Can you work these out from the model? Positions are in its coordinate system, mm. Coordinates: 2 decimals unless noted, no trailing zeros. Order: outer loops, then holes, each group sorted by start corner. A loop starts at its lowest first (then second) coordinate and runs counter-clockwise, first axis right, second up. Notation, with made-up numbers: (85.5, -3.75) -> (122.5, -3.75) arc R20 cw to (122.5, 31.25) -> close; hole circle Ø3 at (52.25, 17.25). An arc over 180 degrees is marked (long way). Return JSON: item names as keys, results as strings. Group by question number.
1) If I drill on probe 1 along Z at (x, y) = (0.55, 0); probe 2 along Z at (x, y) = (0.9, -0.75); probe 3 along Z at (x, y) = (0.4, -9.25), over which ranges is the centre line in solid material (lowest first)? Write a range as from..to.
2) If we section it at C-C, the plane y = 9: Please give me the cut outline in (x, z).
3) For pin 1 (1.8 mm diameter, centred on y = -9, z = 0, fed in from +X), with a flat end and sliding along its axis, tell me the tip position at first contact or that it passes through.
4) If we section it at A-A, the plane z = 0: Please give me the cut outline in (x, y).
from build123d import *

# Parameters (mm, degrees)
F0_R     = 11.5
F1_DEPTH = 1
F2_R     = 1
F3_DEPTH = 1.001


with BuildPart() as f1:
    # F0 (on Right) → F1 (new body)
    with BuildSketch(Plane.YZ):
        Circle(F0_R)
    extrude(amount=F1_DEPTH)

    # F2 (on face) → F3 (cut, through all)
    with BuildSketch(Plane.YZ.offset(1)):
        with Locations((0, 9)):
            Circle(F2_R)
        with Locations((9, 0)):
            Circle(F2_R)
        with Locations((0, -9)):
            Circle(F2_R)
        with Locations((-9, 0)):
            Circle(F2_R)
    extrude(amount=-F3_DEPTH, mode=Mode.SUBTRACT)


solid = f1.part
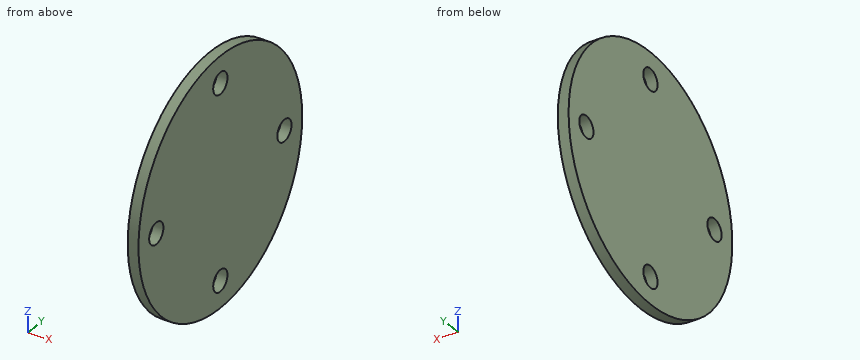
Result sheet:
{
 "1": {"probe 1": "z = -11.5..-10, -8..8, 10..11.5", "probe 2": "z = -11.48..-9.66, -8.34..8.34, 9.66..11.48", "probe 3": "z = -6.83..-0.97, 0.97..6.83"},
 "2": {"outline": "(0, -7.16) -> (1, -7.16) -> (1, -1) -> (0, -1) -> close; (0, 1) -> (1, 1) -> (1, 7.16) -> (0, 7.16) -> close"},
 "3": {"pin 1": "passes through"},
 "4": {"outline": "(0, -11.5) -> (1, -11.5) -> (1, -10) -> (0, -10) -> close; (0, -8) -> (1, -8) -> (1, 8) -> (0, 8) -> close; (0, 10) -> (1, 10) -> (1, 11.5) -> (0, 11.5) -> close"}
}
